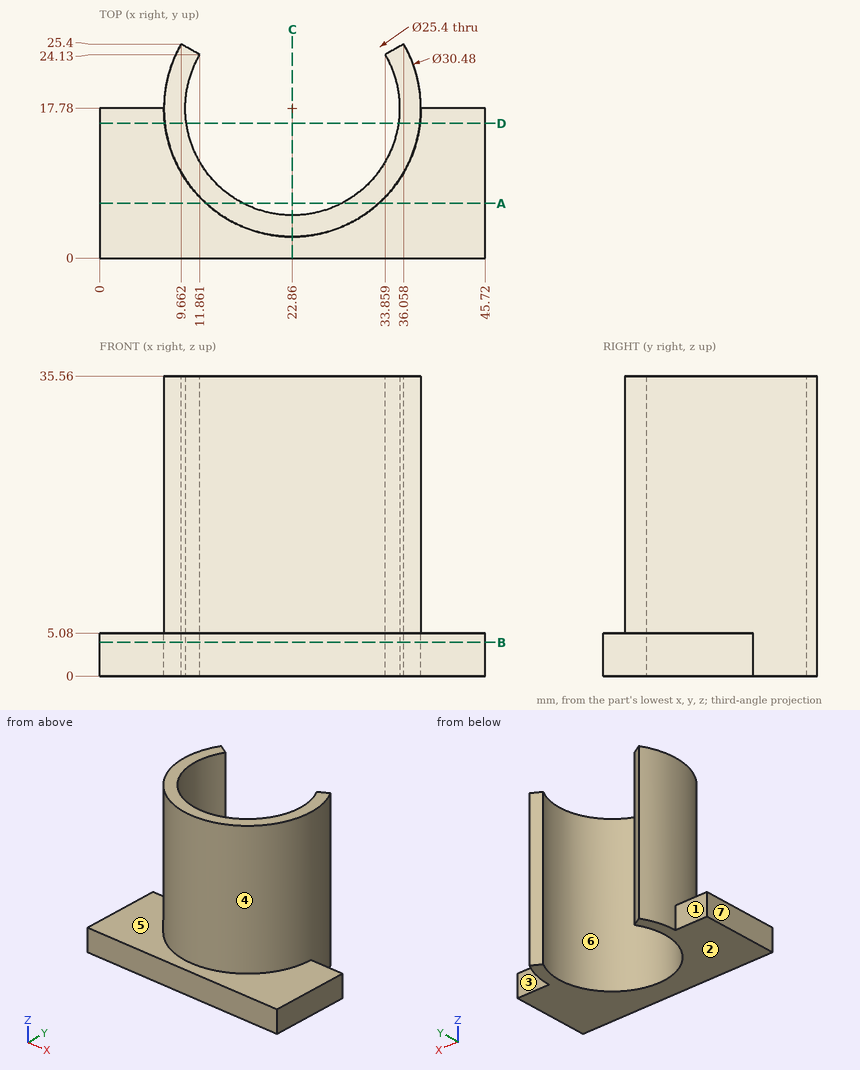
Can you work these out from the drawing? Everything is in mm from the part's minimum corner. A direction names the side the tool comes from. Give positions to 0.01 mm unless a question says otherwise; leave off trailing zeros. Order: outer loops, then holes, each group sorted by start corner. A loop starts at its lowest first (then second) coordinate and runs counter-clockwise, first axis right, second up. Notation, with made-up numbers: M 86.25,25 L 128.25,25 A26 ccw 128.25,63 Z; hole C 81,-9 d4. An arc over 180 degrees is marked long. Write item = value, one per line. Start each with the question number.
Q1. Suppose I cut it at A-A (y = 6.5). Write out the boundary of the cut face in (x, z) (1 decimal).
Q2. Suppose I cut it at D-D (y = 16). Write out the boundary of the cut face in (x, z) (1 decimal).
Q3. Will these pins go through, and if not, where does the flat tip stop? pin 1 Ø4 at (x, z) = (4.5, 3.5) entering from +Y; pin 2 Ø1 at (y, z) = (5.5, 27.5) entering from -X; pin 3 Ø5 at (y, z) = (12, 30.5) entering from -X; pin 4 Ø10 at (x, y) = (28.5, 15.5) entering from +Z.
Q4. Suppose I cut it at B-B (z = 4). Write out the boundary of the cut face in (x, y), plus the area to 3 significant figures.
Q5. Suppose I cut it at C-C (x = 22.86). Write out the boundary of the cut face in (y, z), plus the area to 3 significant figures.
Q6. For the marked faces 1, 2 and 3, which set-ups out of +Z, -Z, +X, -X, +Y, -Y let a thin tool reach every point of the face, with its end or its side?
Q7. We'd pull the mould along X, two halves only. Please class the marked faces 4, 5, 6 and 7: pulls with the +X half, pulls with the -X half, needs draft (parallel to the pull), parting line crosses it, or undercut.
Q8. I need wall thicknesses on probe 1 along X at (y, z) = (17.78, 22); probe 2 along Z at (x, y) = (41, 7.5); probe 3 along Y at (x, z) = (22.86, 14). Which ranges of each line are inside material? Lowest first, please. Write a range as [from, to].
Check result:
q1.outline = M 0,0 L 17,0 L 17,35.6 L 12.6,35.6 L 12.6,5.1 L 0,5.1 Z; M 28.7,0 L 45.7,0 L 45.7,5.1 L 33.1,5.1 L 33.1,35.6 L 28.7,35.6 Z
q2.outline = M 0,0 L 10.3,0 L 10.3,35.6 L 7.7,35.6 L 7.7,5.1 L 0,5.1 Z; M 35.4,0 L 45.7,0 L 45.7,5.1 L 38,5.1 L 38,35.6 L 35.4,35.6 Z
q3.pin_1 = 17.78
q3.pin_2 = 13.19
q3.pin_3 = 7.98
q3.pin_4 = through
q4.outline = M 0,0 L 45.72,0 L 45.72,17.78 L 38.1,17.78 A15.24 ccw 36.06,25.4 L 33.86,24.13 A12.7 cw long 11.86,24.13 L 9.66,25.4 A15.24 ccw 7.62,17.78 L 0,17.78 Z
q4.area = 597 mm2
q5.outline = M 0,0 L 5.08,0 L 5.08,35.56 L 2.54,35.56 L 2.54,5.08 L 0,5.08 Z
q5.area = 103 mm2
q6.face_1 = +Z, -Z, -X, +Y
q6.face_2 = -Z, +X, -X, +Y, -Y
q6.face_3 = +Z, -Z, +X, +Y
q7.face_4 = parting line crosses it
q7.face_5 = needs draft
q7.face_6 = undercut
q7.face_7 = pulls with the -X half
q8.probe_1 = [7.62, 10.16], [35.56, 38.1]
q8.probe_2 = [0, 5.08]
q8.probe_3 = [2.54, 5.08]
